```python
from build123d import *

# Parameters (mm, degrees)
ESQUISSE1_R        = 4
BOSS_EXTRU_1_DEPTH = 3


with BuildPart() as part:
    # Esquisse1 → Boss.-Extru.1 (new body)
    with BuildSketch(Plane.XY):
        with BuildLine():
            Line((-21, 15), (-27.5, 15))
            Line((-27.5, 15), (-27.5, -17.5))
            Line((-27.5, -17.5), (-23.5, -17.5))
            Line((-23.5, -17.5), (-23.5, -15))
            Line((-23.5, -15), (-10.5, -15))
            Line((-10.5, -15), (-10.5, -17.5))
            Line((-10.5, -17.5), (-3.5, -17.5))
            Line((-3.5, -17.5), (-3.5, -15))
            Line((-3.5, -15), (23.5, -15))
            Line((23.5, -15), (23.5, -17.5))
            Line((23.5, -17.5), (27.5, -17.5))
            Line((27.5, -17.5), (27.5, 15))
            Line((27.5, 15), (16, 15))
            Line((16, 15), (16, 17.5))
            Line((16, 17.5), (8, 17.5))
            Line((8, 17.5), (8, 15))
            Line((8, 15), (-5, 15))
            Line((-5, 15), (-5, 17.5))
            Line((-5, 17.5), (-13, 17.5))
            Line((-13, 17.5), (-13, 11))
            ThreePointArc((-13, 11), (-17, 7), (-21, 11))
            Line((-21, 11), (-21, 15))
        make_face()
        with Locations((10, -1.5)):
            Circle(ESQUISSE1_R, mode=Mode.SUBTRACT)
        with Locations((-17, -7.5)):
            Circle(ESQUISSE1_R, mode=Mode.SUBTRACT)
    extrude(amount=BOSS_EXTRU_1_DEPTH)


solid = part.part
```
Verification items for the finished model (mm, model axes). A direction names the side the tool comes from. Round coordinates to 2 decimals unless told otherwise and drop trailing zeros. Loops run counter-clockwise (first coordinate to the right, second up) from the corner with the lowest first, then second, coordinate; pieces in that order, holes last. Notation, with made-up numbers: (40.25, 85) -> (52.25, 85) arc R22 cw to (52.25, 122) -> close; hole circle Ø2 at (-30.75, 77.25). An arc over 180 degrees is marked (long way). Answer as a JSON object with one key per item and string values.
Q1. Scan lines: line 1 (Y direction, x = 10, z = 2.05); line 2 (X direction, y = 12.5, z = 0.6); line 3 (Y direction, x = 5.5, z = 2.3). Record each from-to range of solid material in increasing order. Write a range as from..to.
Data:
{"line 1": "y = -15..-5.5, 2.5..17.5", "line 2": "x = -27.5..-21, -13..27.5", "line 3": "y = -15..15"}
Q2. Go/stop test with flat-tipped pins: P1, Ø1.2, axis at y = 16, z = 1, coming from the -X side; P2, Ø0.9, axis at x = 1.5, z = 2, coming from the +Y side. Record where each tip stops, or that it passes through.
Data:
{"P1": "stops at x = -13", "P2": "stops at y = 15"}
Q3. Access from +Z, -Z, +X, -X, +Y, -Y to the whole of each face (thin tool, end or side, straight path). Record for faces 1 (the flat face through (-24, 15, 1)), 2 (the flat face through (23.5, -16, 1)), 3 (the flat face through (-13, 14, 1)).
Data:
{"face 1": "+Z, -Z, -X, +Y", "face 2": "+Z, -Z, -Y", "face 3": "+Z, -Z, +Y"}
Q4. Section check C-C (z = 1.9). Record the boundary of the cut face in (x, y), then the cut area to 3 significant figures.
Data:
{"outline": "(-27.5, -17.5) -> (-23.5, -17.5) -> (-23.5, -15) -> (-10.5, -15) -> (-10.5, -17.5) -> (-3.5, -17.5) -> (-3.5, -15) -> (23.5, -15) -> (23.5, -17.5) -> (27.5, -17.5) -> (27.5, 15) -> (16, 15) -> (16, 17.5) -> (8, 17.5) -> (8, 15) -> (-5, 15) -> (-5, 17.5) -> (-13, 17.5) -> (-13, 11) arc R4 cw to (-21, 11) -> (-21, 15) -> (-27.5, 15) -> close; hole circle Ø8 at (-17, -7.5); hole circle Ø8 at (10, -1.5)", "area": "1,570 mm2"}
Q5. Section check B-B (y = 12). Record the boundary of the cut face in (x, z), then the cut area to 3 significant figures.
Data:
{"outline": "(-27.5, 0) -> (-21, 0) -> (-21, 3) -> (-27.5, 3) -> close; (-13, 0) -> (27.5, 0) -> (27.5, 3) -> (-13, 3) -> close", "area": "141 mm2"}
Q6. Draft check along X on faces 4 (the flat face through (16, 16, 1)), 5 (the flat face through (2, 15, 1)), 6 (the flat face through (0, 0, 3)), 7 (the flat face through (-23.5, -16, 1)). Enter one of: pulls with the +X half, pulls with the -X half, needs draft (parallel to the pull), parting line crosses it, or undercut.
Data:
{"face 4": "pulls with the +X half", "face 5": "undercut", "face 6": "needs draft", "face 7": "undercut"}
Q7. Section check A-A (x = 10). Record the boundary of the cut face in (y, z), then the cut area to 3 significant figures.
Data:
{"outline": "(-15, 0) -> (-5.5, 0) -> (-5.5, 3) -> (-15, 3) -> close; (2.5, 0) -> (17.5, 0) -> (17.5, 3) -> (2.5, 3) -> close", "area": "73.5 mm2"}
